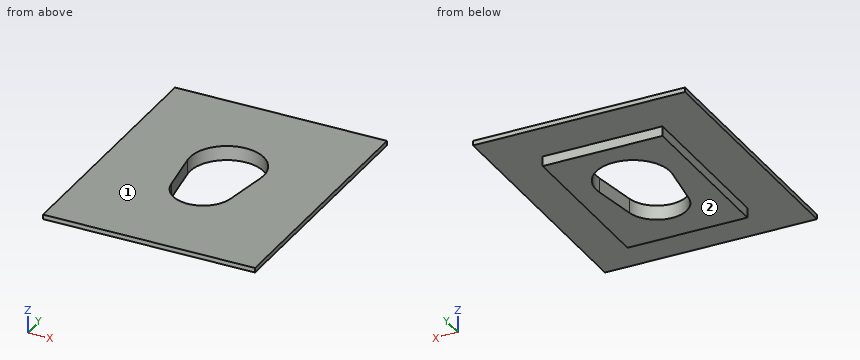
```python
from build123d import *

# Parameters (mm, degrees)
SKETCH1_W           = 26
SKETCH1_H           = 36
BOSS_EXTRUDE1_DEPTH = 1.5625
SKETCH2_W           = 46
SKETCH2_H           = 56
SKETCH2_W_2         = 26
SKETCH2_H_2         = 36
BOSS_EXTRUDE2_DEPTH = 1


with BuildPart() as part:
    # Sketch1 → Boss-Extrude1 (new, symmetric)
    with BuildSketch(Plane.XY):
        with Locations((0, 5)):
            Rectangle(SKETCH1_W, SKETCH1_H)
        with BuildLine():
            Line((-6.426458978, -0.975), (-7.909487973, 8.8))
            ThreePointArc((-7.909487973, 8.8), (0, 18), (7.909487973, 8.8))
            Line((7.909487973, 8.8), (6.426458978, -0.975))
            ThreePointArc((6.426458978, -0.975), (0, -6.5), (-6.426458978, -0.975))
        make_face(mode=Mode.SUBTRACT)
    extrude(amount=BOSS_EXTRUDE1_DEPTH, both=True)

    # Sketch2 → Boss-Extrude2 (add)
    with BuildSketch(Plane(origin=(0, 0, 1.5625), x_dir=(-1, 0, 0), z_dir=(0, 0, -1))):
        with Locations((0, 5)):
            Rectangle(SKETCH2_W, SKETCH2_H)
        with Locations((0, 5)):
            Rectangle(SKETCH2_W_2, SKETCH2_H_2, mode=Mode.SUBTRACT)
    extrude(amount=BOSS_EXTRUDE2_DEPTH)


solid = part.part
```
Work out the finished part from the listing and answer in its coordinate system (mm). Face numbers are marked on the shaded views. Give positions to 0.01 mm unless a question says otherwise; leave off trailing zeros. Order: outer loops, then holes, each group sorted by start corner. A loop starts at its lowest first (then second) coordinate and runs counter-clockwise, first axis right, second up.
1. The mould has two halves that part along Z. Classify the marked faces 1 and 2: released by +Z, released by -Z, zero draft, split by the parting line, or undercut.
Result sheet:
face 1: released by +Z
face 2: released by -Z
2. Section C-C, the plane y = 20.5 is taken. Determine the outline of the cut face in (x, z), and give its area (3 significant figures).
Result sheet:
outline: (-23, 0.56) - (-13, 0.56) - (-13, -1.56) - (13, -1.56) - (13, 0.56) - (23, 0.56) - (23, 1.56) - (-23, 1.56) - close
area: 101 mm2
3. Straight lines are drawn through the part: L1, parallel to Y at x = 0, z = 0.8; L2, parallel to Y at x = 0, z = 0.35; L3, parallel to X at y = 10, z = 0.1. For each, find the intervals that lie inside material, in ascending order.
Result sheet:
L1: y = -23 to -6.5, 18 to 33
L2: y = -13 to -6.5, 18 to 23
L3: x = -13 to -8, 8 to 13
4. Section B-B, the plane y = 10 is taken. Determine the outline of the cut face in (x, z).
Result sheet:
outline: (-23, 0.56) - (-13, 0.56) - (-13, -1.56) - (-8, -1.56) - (-8, 1.56) - (-23, 1.56) - close; (8, -1.56) - (13, -1.56) - (13, 0.56) - (23, 0.56) - (23, 1.56) - (8, 1.56) - close
5. Each of these flat-tipped pins is pushed along its axis until it touches: P1, Ø9.5, axis at x = 0, y = 10, coming from the -Z side (3 decimals); P2, Ø1.7, axis at y = 13.5, z = -0.5, coming from the -X side; P3, Ø1.1, axis at x = 3, z = -0.5, coming from the -Y side; P4, Ø1.7, axis at y = -0.5, z = 0, coming from the +X side. Where does it stop, or does it pass through?
Result sheet:
P1: passes through
P2: stops at x = -13
P3: stops at y = -13
P4: stops at x = 23
6. Section D-D, the plane z = -0.75 is taken. Determine the outline of the cut face in (x, y) (3 decimals), and give its area (3 significant figures).
Result sheet:
outline: (-13, -13) - (13, -13) - (13, 23) - (-13, 23) - close; hole (-7.909, 8.8) - (-6.426, -0.975) arc R6.5 ccw to (6.426, -0.975) - (7.909, 8.8) arc R8 ccw (long way) to start
area: 622 mm2
7. Section A-A, the plane x = 0 is taken. Determine the outline of the cut face in (y, z).
Result sheet:
outline: (-23, 0.56) - (-13, 0.56) - (-13, -1.56) - (-6.5, -1.56) - (-6.5, 1.56) - (-23, 1.56) - close; (18, -1.56) - (23, -1.56) - (23, 0.56) - (33, 0.56) - (33, 1.56) - (18, 1.56) - close
